```python
from build123d import *

# Parameters (mm, degrees)
SKETCH1_R                       = 34.25
SKETCH1_R_2                     = 32.5
BULK_DEPTH                      = 500
SKETCH2_R                       = 1.75
LAUNCH_LUG_SCREW_HOLES_DEPTH    = 503.340646375
SKETCH3_W                       = 6.5
SKETCH3_H                       = 120
THRU_WALL_FIN_CUTS_DEPTH        = 503.340646488
THRU_WALL_FIN_CUT_PATTERN_COUNT = 2
THRU_WALL_FIN_CUT_PATTERN_ANGLE = 90


with BuildPart() as part:
    # Sketch1 → BULK (new body)
    with BuildSketch(Plane(origin=(0, 0, 0), x_dir=(1, 0, 0), z_dir=(0, 1, 0))):
        with Locations(Location((0, 0, 0), (0, 0, 270))):
            Circle(SKETCH1_R)
        with Locations(Location((0, 0, 0), (0, 0, 270))):
            Circle(SKETCH1_R_2, mode=Mode.SUBTRACT)
    extrude(amount=BULK_DEPTH)

    # Sketch2 → LAUNCH LUG SCREW HOLES (cut, through all)
    with BuildSketch(Plane(origin=(0, 0, 0), x_dir=(0.7071067811865477, 0, 0.7071067811865475), z_dir=(-0.7071067811865475, 0, 0.7071067811865477))):
        with Locations(Location((0, 25, 0), (0, 0, 180))):
            Circle(SKETCH2_R)
        with Locations(Location((0, 450, 0), (0, 0, 180))):
            Circle(SKETCH2_R)
    extrude(amount=LAUNCH_LUG_SCREW_HOLES_DEPTH, mode=Mode.SUBTRACT)

    # Sketch3 → THRU WALL FIN CUTS (cut, symmetric)
    with BuildSketch(Plane.XY):
        with Locations((0, 70)):
            Rectangle(SKETCH3_W, SKETCH3_H)
    thru_wall_fin_cuts = extrude(amount=THRU_WALL_FIN_CUTS_DEPTH, both=True, mode=Mode.SUBTRACT)

    # THRU WALL FIN CUT PATTERN: THRU WALL FIN CUTS ×2 about axis
    thru_wall_fin_cut_pattern_axis = Axis((0, -25, 0), (0, 1, 0))
    for i in range(1, THRU_WALL_FIN_CUT_PATTERN_COUNT):
        add(thru_wall_fin_cuts.rotate(thru_wall_fin_cut_pattern_axis, i * THRU_WALL_FIN_CUT_PATTERN_ANGLE / (THRU_WALL_FIN_CUT_PATTERN_COUNT - 1)), mode=Mode.SUBTRACT)


solid = part.part
```
The model under review builds one solid part; all positions refer to its coordinate system, in mm. Round coordinates to 2 decimals unless told otherwise and drop trailing zeros. Loops run counter-clockwise (first coordinate to the right, second up) from the corner with the lowest first, then second, coordinate; pieces in that order, holes last. Notation, with made-up numbers: (48, -1) - (84, -1) arc R23 cw to (84, 11) - close; hole circle Ø3 at (89, 67.25). An arc over 180 degrees is marked (long way). Use a Markdown table: item, result. Add a question column.
Q1. For probe 1 along Z at (x, y) = (0, 232); probe 2 along X at (y, z) = (213, 4), list the stretches that pass through material, from the lowest coordinate up.
Q2. Add section B-B (z = 13). State the section outline as (x, y) points.
Q3. Add section D-D (y = 325.5). State the section outline as (x, z) points.
Q4. Add section C-C (x = 23). State the section outline as (y, z) points, plus the area to 3 significant figures.
Q5. The part is to be moulded in two halves that separate along X. For faces 1 (the face through (10.288, 246.5, 32.668)), 2 (the face through (26, 500, 20)), 3 (the face through (9.76, 246.5, 31)), say which applies: pulls with the +X half, pulls with the -X half, needs draft (parallel to the pull), parting line crosses it, or undercut.
Q6. Insertion check: pin 1 Ø2 at (x, z) = (-27, -13) entering from -Y; pin 2 Ø0.6 at (x, z) = (-34, 0) entering from -Y; pin 3 Ø4 at (y, z) = (310.5, -14) entering from +X; pin 4 Ø12 at (x, y) = (-14.5, 271) entering from -Z. Each pin has a flat end and moves straight along its axis. Give the tip position at first contact, or say it passes through.
Q7. Add section A-A (y = 102.5). State the section outline as (x, z) points, plus the area to 3 significant figures.
Worked answers:
| question | item | result |
|---|---|---|
| 1 | probe 1 | -34.25 to -32.5, 32.5 to 34.25 |
| 1 | probe 2 | -34.02 to -32.25, 32.25 to 34.02 |
| 2 | outline | (-31.69, 0) - (-29.79, 0) - (-29.79, 500) - (-31.69, 500) - close; (29.79, 0) - (31.69, 0) - (31.69, 500) - (29.79, 500) - close |
| 3 | outline | circle Ø68.5 at (0, 0); hole circle Ø65 at (0, 0) |
| 4 | outline | (0, -25.38) - (500, -25.38) - (500, -22.96) - (0, -22.96) - close; (0, 22.96) - (500, 22.96) - (500, 25.38) - (0, 25.38) - close |
| 4 | area | 2,420 mm² |
| 5 | face 1 | parting line crosses it |
| 5 | face 2 | needs draft |
| 5 | face 3 | undercut |
| 6 | pin 1 | through |
| 6 | pin 2 | y = 0 |
| 6 | pin 3 | x = 32.08 |
| 6 | pin 4 | z = -33.18 |
| 7 | outline | (-34.1, -3.25) arc R34.25 ccw to (-3.25, -34.1) - (-3.25, -32.34) arc R32.5 cw to (-32.34, -3.25) - close; (-34.1, 3.25) - (-32.34, 3.25) arc R32.5 cw to (-3.25, 32.34) - (-3.25, 34.1) arc R34.25 ccw to start; (3.25, -34.1) arc R34.25 ccw to (34.1, -3.25) - (32.34, -3.25) arc R32.5 cw to (3.25, -32.34) - close; (3.25, 32.34) arc R32.5 cw to (32.34, 3.25) - (34.1, 3.25) arc R34.25 ccw to (3.25, 34.1) - close |
| 7 | area | 321 mm² |
